from build123d import *

# Parameters (mm, degrees)
SKETCH1_W           = 40
SKETCH1_H           = 40
BOSS_EXTRUDE1_DEPTH = 40
CUT_EXTRUDE1_DEPTH  = 40
SKETCH3_W           = 20
SKETCH3_H           = 20
CUT_EXTRUDE2_DEPTH  = 40
CUT_EXTRUDE4_DEPTH  = 40
CUT_EXTRUDE5_DEPTH  = 20


with BuildPart() as part:
    # Sketch1 → Boss-Extrude1 (new body)
    with BuildSketch(Plane.XY):
        with Locations((20, 20)):
            Rectangle(SKETCH1_W, SKETCH1_H)
    extrude(amount=BOSS_EXTRUDE1_DEPTH)

    # Sketch2 → Cut-Extrude1 (cut)
    with BuildSketch(Plane.XY.offset(40)):
        Polygon((40, 40), (0, 40), (0, 20), align=None)
    extrude(amount=-CUT_EXTRUDE1_DEPTH, mode=Mode.SUBTRACT)

    # Sketch3 → Cut-Extrude2 (cut)
    with BuildSketch(Plane(origin=(40, 0, 0), x_dir=(0, 0, -1), z_dir=(1, 0, 0))):
        with Locations((-30, 30)):
            Rectangle(SKETCH3_W, SKETCH3_H)
    extrude(amount=-CUT_EXTRUDE2_DEPTH, mode=Mode.SUBTRACT)

    # Sketch4 → Cut-Extrude4 (cut)
    with BuildSketch(Plane.XY.offset(40)):
        Polygon((0, 20), (20, 0), (0, 0), align=None)
    extrude(amount=-CUT_EXTRUDE4_DEPTH, mode=Mode.SUBTRACT)

    # Sketch5 → Cut-Extrude5 (cut)
    with BuildSketch(Plane(origin=(40, 0, 0), x_dir=(0, 0, -1), z_dir=(1, 0, 0))):
        Polygon((-20, 20), (-40, 0), (-40, 20), align=None)
    extrude(amount=-CUT_EXTRUDE5_DEPTH, mode=Mode.SUBTRACT)


solid = part.part
Verification items for the finished model (mm, model axes). A direction names the side the tool comes from. Coordinates: 2 decimals unless noted, no trailing zeros. Write each loop counter-clockwise with the first axis right and the second up, starting at its lowest first coordinate (ties: lowest second). Pieces come first, ordered by that corner, then holes. Notation, with made-up numbers: (39.5, -18.5) -> (75.5, -18.5) arc R31 cw to (75.5, 5.5) -> close; hole circle Ø11 at (1, 87.25). An arc over 180 degrees is marked (long way). One line per item, written item: value. Start each with the question number.
Q1. Cross-section at B-B on z = 32.5. Enter the section's corners in (x, y).
Q2. Thickness scan on L1, parallel to Z at x = 28, y = 26.5; L2, parallel to X at y = 7, z = 10; L3, parallel to X at y = 35, z = 12. Record the ranges inside material, lowest first. Write a range as from..to.
Q3. Cross-section at C-C on y = 36. Enter the section's corners in (x, z).
Q4. Access from +Z, -Z, +X, -X, +Y, -Y to the whole of each face (thin tool, end or side, straight path). Record for faces 1 (the flat face through (10, 10, 20)), 2 (the flat face through (25, 28, 20)), 3 (the flat face through (20, 15, 34)).
Q5. Cross-section at D-D on x = 34. Enter the section's corners in (y, z), and give its area (3 significant figures).
Q6. Cross-section at A-A on x = 5.5. Enter the section's corners in (y, z), and give its area (3 significant figures).
Q7. Go/stop test with flat-tipped pins: P1, Ø5, axis at x = 28, z = 4.5, coming from the -Y side; P2, Ø12, axis at y = 12.5, z = 30.5, coming from the -X side; P3, Ø16, axis at x = 9.5, z = 32.5, coming from the +Y side; P4, Ø10, axis at x = 16, y = 28, coming from the +Z side. Record where each tip stops, or that it passes through.
Checked values:
1. outline: (0, 20) -> (20, 0) -> (40, 0) -> (40, 7.5) -> (20, 7.5) -> (20, 20) -> close
2. L1: z = 0..20
2. L2: x = 13..40
2. L3: x = 30..40
3. outline: (32, 0) -> (40, 0) -> (40, 20) -> (32, 20) -> close
4. face 1: +Z, -Z, -X, -Y
4. face 2: +Z, +X, -X, +Y
4. face 3: +Z, +X, +Y
5. outline: (0, 0) -> (37, 0) -> (37, 20) -> (20, 20) -> (0, 40) -> close
5. area: 940 mm²
6. outline: (14.5, 0) -> (22.75, 0) -> (22.75, 20) -> (20, 20) -> (20, 40) -> (14.5, 40) -> close
6. area: 275 mm²
7. P1: stops at y = 0
7. P2: stops at x = 1.5
7. P3: stops at y = 20
7. P4: stops at z = 20
